```python
from build123d import *

# Parameters (mm, degrees)
F1_DEPTH = 12
F2_R     = 5
F3_R     = 5
F5_DEPTH = 50.001


with BuildPart() as f1:
    # F0 (on Top) → F1 (new body)
    with BuildSketch(Plane.XY):
        Polygon((-54.5071489434, 162.6097643375), (-67.0071489434, 162.6097643375), (-67.0071489434, -167.3902356625), (-54.5071489434, -167.3902356625), (-54.5071489434, -154.3902356625), (-29.5071489434, -154.3902356625), (-29.5071489434, -167.3902356625), (-17.0071489434, -167.3902356625), (-17.0071489434, 162.6097643375), (-29.5071489434, 162.6097643375), (-29.5071489434, 149.6097643375), (-54.5071489434, 149.6097643375), align=None)
    extrude(amount=F1_DEPTH)

    # F2
    f2_edges = [f1.edges().sort_by_distance(p)[0] for p in [
        (-67.007149, 162.609764, 6),
    ]]
    fillet(f2_edges, radius=F2_R)

    # F3
    f3_edges = [f1.edges().sort_by_distance(p)[0] for p in [
        (-67.007149, -167.390236, 6),
        (-17.007149, -167.390236, 6),
        (-17.007149, 162.609764, 6),
    ]]
    fillet(f3_edges, radius=F3_R)

    # F4 (on face) → F5 (cut, through all)
    with BuildSketch(Plane.YZ.offset(-17.0071489434)):
        with BuildLine():
            Line((157.6097643375, 3), (157.6097643375, 9))
            ThreePointArc((157.6097643375, 9), (154.6097643375, 6), (157.6097643375, 3))
        make_face()
        with BuildLine():
            ThreePointArc((160.6097643375, 6), (159.7310846811, 8.1213203436), (157.6097643375, 9))
            Line((157.6097643375, 9), (157.6097643375, 3))
            ThreePointArc((157.6097643375, 3), (159.7310846811, 3.8786796564), (160.6097643375, 6))
        make_face()
        with BuildLine():
            Line((-162.3902356625, 3), (-162.3902356625, 9))
            ThreePointArc((-162.3902356625, 9), (-165.3902356625, 6), (-162.3902356625, 3))
        make_face()
        with BuildLine():
            ThreePointArc((-162.3902356625, 3), (-160.2689153189, 3.8786796564), (-159.3902356625, 6))
            ThreePointArc((-159.3902356625, 6), (-160.2689153189, 8.1213203436), (-162.3902356625, 9))
            Line((-162.3902356625, 9), (-162.3902356625, 3))
        make_face()
    extrude(amount=-F5_DEPTH, mode=Mode.SUBTRACT)


solid = f1.part
```
Can you work these out from the model? Positions are in its coordinate system, mm. A direction names the side the tool comes from. Coordinates: 2 decimals unless noted, no trailing zeros. Order: outer loops, then holes, each group sorted by start corner. A loop starts at its lowest first (then second) coordinate and runs counter-clockwise, first axis right, second up.
1. I need wall thicknesses on line 1 (Y direction, x = -21, z = 7); line 2 (Y direction, x = -56.5, z = 6.75); line 3 (Y direction, x = -49, z = 6). Which ranges of each line are inside material? Lowest first, please.
2. For faces 1 (the face through (-67.007, 0, 6)), 2 (the face through (-29.507, -159, 6)), 3 (the face through (-42, 149.61, 6)), which set-ups out of +Z, -Z, +X, -X, +Y, -Y let a thin tool reach every point of the face, with its end or its side?
3. If we section it at A-A (x = -34): Please give me the cut outline in (y, z), then the cut area to 3 significant figures.
Entries:
1. line 1: y = -167.29 to -165.22, -159.56 to 154.78, 160.44 to 162.51
1. line 2: y = -167.39 to -165.29, -159.49 to 154.71, 160.51 to 162.61
1. line 3: y = -154.39 to 149.61
2. face 1: +Z, -Z, -X, +Y, -Y
2. face 2: +Z, -Z, -Y
2. face 3: +Z, -Z, +Y
3. outline: (-154.39, 0) - (149.61, 0) - (149.61, 12) - (-154.39, 12) - close
3. area: 3,650 mm2
